Model file for the job. Use its own axes, mm. A direction names the side the tool comes from. Give positions to 0.01 mm unless a question says otherwise; leave off trailing zeros. Loops run counter-clockwise (first coordinate to the right, second up) from the corner with the lowest first, then second, coordinate; pieces in that order, holes last. Notation, with made-up numbers: M 44,-2.75 L 63,-2.75 A9 ccw 63,11.25 Z; hole C 33.25,49.25 d10. An arc over 180 degrees is marked long. Answer in a Markdown table with one row per item.
```python
from build123d import *


with BuildPart() as part:
    # Sketch → Revolution (revolve)
    with BuildSketch(Plane.XZ):
        Polygon((0.040665, 0), (0.040665, 27.5), (2.740665, 27.5), (2.740665, 25), (31.540664, 25), (34.540664, 22.8), (34.540664, 22.3), (2.740665, 22.3), (2.740665, 0), align=None)
    revolve(axis=Axis((0, 0, 0), (1, 0, 0)))


solid = part.part
```
Q1. Saw through at A-A (z = 0). Give the cut face in (x, y).
Reported:
| item | result |
|---|---|
| outline | M 0.04,-27.5 L 2.74,-27.5 L 2.74,-25 L 31.54,-25 L 34.54,-22.8 L 34.54,-22.3 L 2.74,-22.3 L 2.74,22.3 L 34.54,22.3 L 34.54,22.8 L 31.54,25 L 2.74,25 L 2.74,27.5 L 0.04,27.5 Z |
Q2. Drop flat-ended pins along their axis: pin 1 (2 mm diameter, centred on x = 26.5, z = 8.5, fed in from +Y); pin 2 (12 mm diameter, centred on x = 28.5, y = -17, fed in from -Z); pin 3 (16.5 mm diameter, centred on y = 0, z = -0.5, fed in from +X). Give the stop position or say it passes through.
Reported:
| item | result |
|---|---|
| pin 1 | y = 23.85 |
| pin 2 | z = -22.45 |
| pin 3 | x = 2.74 |
Q3. Probe probe 1 along Y at (x, z) = (15, 0); probe 2 along X at (y, z) = (-14.5, -5); probe 3 along Y at (x, z) = (8.5, -4.5). List the from-to ranges inside material, lowest first.
Reported:
| item | result |
|---|---|
| probe 1 | -25 to -22.3, 22.3 to 25 |
| probe 2 | 0.04 to 2.74 |
| probe 3 | -24.59 to -21.84, 21.84 to 24.59 |
Q4. Mould opens along Z. For faces 3 (the face through (18.42, -6.7, 21.27)), 4 (the face through (1.41, 26.846, -5.961)), 5 (the face through (34.541, 22, 5)) say: released by +Z, released by -Z, zero draft, split by the parting line, or undercut.
Reported:
| item | result |
|---|---|
| face 3 | undercut |
| face 4 | split by the parting line |
| face 5 | zero draft |
Q5. 3-axis set-ups, long thin cutter, end or side, ignore diameter. For faces 1 (the face through (17.342, -7.509, 23.846)), 2 (the face through (0.041, 0, 0)): which of +Z, -Z, +X, -X, +Y, -Y reach the whole face in a straight line?
Reported:
| item | result |
|---|---|
| face 1 | +X |
| face 2 | +Z, -Z, -X, +Y, -Y |
Q6. Saw through at C-C (x = 7). Give the cut face in (y, z).
Reported:
| item | result |
|---|---|
| outline | C 0,0 d50; hole C 0,0 d44.6 |
